Verification items for the finished model (mm, model axes). Face numbers are marked on the shaded views. Give positions to 0.01 mm unless a question says otherwise; leave off trailing zeros. Order: outer loops, then holes, each group sorted by start corner. A loop starts at its lowest first (then second) coordinate and runs counter-clockwise, first axis right, second up.
(1) Scan lines: L1, parallel to Y at x = 1.5, z = -17.5; L2, parallel to Z at x = 6.5, y = 4.5; L3, parallel to Z at x = 2.75, y = 6.25. Record each from-to range of solid material in increasing order.
(2) Sectioned sample at D-D on y = 3.5. Record the cut outline in (x, z), plus the area to 3 significant figures.
(3) Sectioned sample at C-C on y = 7.25. Record the cut outline in (x, z).
(4) Gauge pin test, flat end, axial feed: pin 1 (2.5 mm diameter, centred on y = 6, z = -17.5, fed in from -X). Record the tip position at first contact, or that the pin passes through.
(5) Mould release check, pull along Z, two halves, no side actions. Record for the marked faces 1, 2 and 3: pulls with the +Z half, pulls with the -Z half, needs draft (parallel to the pull), parting line crosses it, or undercut.
(6) Sectioned sample at A-A on z = -17.5. Record the cut outline in (x, y).
(7) Sectioned sample at B-B on x = 5.5. Record the cut outline in (y, z), plus the area to 3 significant figures.
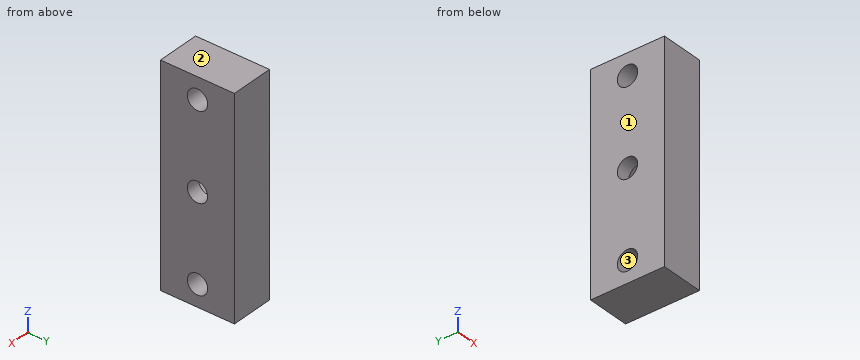
```python
from build123d import *

# Parameters (mm, degrees)
SKETCH1_W           = 35
SKETCH1_H           = 12
SKETCH1_R           = 1.65
BOSS_EXTRUDE1_DEPTH = 7
CUT_EXTRUDE1_START  = -2.25
CUT_EXTRUDE1_DEPTH  = 2.5


with BuildPart() as part:
    # Sketch1 → Boss-Extrude1 (new body)
    with BuildSketch(Plane(origin=(0, 0, 0), x_dir=(0, 0, -1), z_dir=(1, 0, 0))):
        with Locations((17.5, 6)):
            Rectangle(SKETCH1_W, SKETCH1_H)
        with Locations((3.5, 6)):
            Circle(SKETCH1_R, mode=Mode.SUBTRACT)
        with Locations((31.5, 6)):
            Circle(SKETCH1_R, mode=Mode.SUBTRACT)
        with Locations((17.5, 6)):
            Circle(SKETCH1_R, mode=Mode.SUBTRACT)
    extrude(amount=BOSS_EXTRUDE1_DEPTH)

    # Sketch2 → Cut-Extrude1 (cut)
    with BuildSketch(Plane(origin=(7, 0, 0), x_dir=(0, 0, -1), z_dir=(1, 0, 0)).offset(CUT_EXTRUDE1_START)):
        Polygon((20.790896534, 6), (19.145448267, 8.85), (15.854551733, 8.85), (14.209103466, 6), (15.854551733, 3.15), (19.145448267, 3.15), align=None)
    extrude(amount=-CUT_EXTRUDE1_DEPTH, mode=Mode.SUBTRACT)


solid = part.part
```
Ans:
1. L1: y = 0 to 4.35, 7.65 to 12
1. L2: z = -35 to -32.19, -30.81 to -18.19, -16.81 to -4.19, -2.81 to 0
1. L3: z = -35 to -33.13, -29.87 to -20.65, -14.35 to -5.13, -1.87 to 0
2. outline: (0, -35) - (7, -35) - (7, 0) - (0, 0) - close; hole (2.25, -19.35) - (4.75, -19.35) - (4.75, -15.65) - (2.25, -15.65) - close
2. area: 236 mm2
3. outline: (0, -35) - (7, -35) - (7, -32.58) - (0, -32.58) - close; (0, -30.42) - (7, -30.42) - (7, -18.58) - (4.75, -18.58) - (4.75, -20.07) - (2.25, -20.07) - (2.25, -18.58) - (0, -18.58) - close; (0, -16.42) - (2.25, -16.42) - (2.25, -14.93) - (4.75, -14.93) - (4.75, -16.42) - (7, -16.42) - (7, -4.58) - (0, -4.58) - close; (0, -2.42) - (7, -2.42) - (7, 0) - (0, 0) - close
4. pin 1: passes through
5. face 1: needs draft
5. face 2: pulls with the +Z half
5. face 3: undercut
6. outline: (0, 0) - (7, 0) - (7, 4.35) - (4.75, 4.35) - (4.75, 3.15) - (2.25, 3.15) - (2.25, 4.35) - (0, 4.35) - close; (0, 7.65) - (2.25, 7.65) - (2.25, 8.85) - (4.75, 8.85) - (4.75, 7.65) - (7, 7.65) - (7, 12) - (0, 12) - close
7. outline: (0, -35) - (12, -35) - (12, 0) - (0, 0) - close; hole circle Ø3.3 at (6, -31.5); hole circle Ø3.3 at (6, -17.5); hole circle Ø3.3 at (6, -3.5)
7. area: 394 mm2
